from build123d import *

# Parameters (mm, degrees)
SKETCH025_W     = 41
SKETCH025_H     = 41
PAD017_DEPTH    = 22.6
SKETCH026_R     = 19.8
PAD018_DEPTH    = 12.6
SKETCH027_W     = 9
SKETCH027_H     = 4.7
POCKET007_DEPTH = 5


with BuildPart() as part:
    # Sketch025 → Pad017 (new body)
    with BuildSketch(Plane.XY):
        with Locations((3.199544, 3.041725)):
            Rectangle(SKETCH025_W, SKETCH025_H)
    extrude(amount=PAD017_DEPTH)

    # Sketch026 (on Face6 of Pad017) → Pad018 (join)
    with BuildSketch(Plane.XY.offset(22.6)):
        with Locations((3.297032, 2.892403)):
            Circle(SKETCH026_R)
    extrude(amount=PAD018_DEPTH)

    # Sketch027 (on Face3 of Pad018) → Pocket007 (cut)
    with BuildSketch(Plane.XZ.offset(17.458275)):
        with Locations((3.457133, 7.14271)):
            Rectangle(SKETCH027_W, SKETCH027_H)
    extrude(amount=-POCKET007_DEPTH, mode=Mode.SUBTRACT)


with BuildPart() as part_1:
    # Body006 placement: moved
    add(part.part.moved(Location((-5, 10, 65))))


solid = part_1.part
The model under review builds one solid part; all positions refer to its coordinate system, in mm. A direction names the side the tool comes from. Round coordinates to 2 decimals unless told otherwise and drop trailing zeros. Order: outer loops, then holes, each group sorted by start corner. A loop starts at its lowest first (then second) coordinate and runs counter-clockwise, first axis right, second up. Notation, with made-up numbers: (41, 76.25) -> (80, 76.25) arc R10 ccw to (80, 94.25) -> close; hole circle Ø1 at (4, 47.5). An arc over 180 degrees is marked (long way). Write item = value, one per line. Start each with the question number.
Item 1: Consider section C-C on x = 1.5. Write out the cut boundary in (y, z), plus the area to 3 significant figures.
Item 2: For line 1 along Z through (x, y) = (-4.5, -5); line 2 along Z through (x, y) = (17.5, 31); line 3 along Y through (x, z) = (-0.5, 73), list the stretches that pass through material, from the lowest coordinate up.
Item 3: Mouldability with a two-part tool opening along X and no side actions: class faces 4 (the face through (2.957, -5, 72)), 5 (the face through (-2, 13, 65)), 6 (the face through (18.7, 13, 76)) as released by +X, released by -X, zero draft, split by the parting line, or undercut.
Item 4: Clearance check with flat-ended pins moving along their axes: pin 1 Ø1.5 at (y, z) = (19, 88.5) entering from -X; pin 2 Ø1.5 at (x, z) = (-3.5, 93.5) entering from -Y; pin 3 Ø1 at (y, z) = (20, 88.5) entering from -X. State where each tip first meets the part, or that it passes through.
Item 5: Consider section A-A on z = 71. Write out the cut boundary in (x, y).
Item 6: Consider section B-B on y = 8.5. Write out the cut boundary in (x, z).
Item 7: Consider section D-D on z = 91. Write out the cut boundary in (x, y), plus the area to 3 significant figures.
Item 8: For faces 1 (the face through (-2, -5, 74.493)), 2 (the face through (-9.5, 31.4, 87.6)), 3 (the face through (-2, -7.458, 76)), list the 3-axis set-ups (+Z, -Z, +X, -X, +Y, -Y) from which the entire face can be reached by the end or side of a thin tool; tool diameter is ignored.
Conclusion:
q1.outline = (-7.46, 65) -> (33.54, 65) -> (33.54, 87.6) -> (32.43, 87.6) -> (32.43, 100.2) -> (-6.65, 100.2) -> (-6.65, 87.6) -> (-7.46, 87.6) -> (-7.46, 74.49) -> (-2.46, 74.49) -> (-2.46, 69.79) -> (-7.46, 69.79) -> close
q1.area = 1,400 mm2
q2.line_1 = 65 to 69.79, 74.49 to 100.2
q2.line_2 = 65 to 87.6
q2.line_3 = -2.46 to 33.54
q3.face_4 = undercut
q3.face_5 = zero draft
q3.face_6 = released by +X
q4.pin_1 = -20.76
q4.pin_2 = -6.88
q4.pin_3 = -20.37
q5.outline = (-22.3, -7.46) -> (-6.04, -7.46) -> (-6.04, -2.46) -> (2.96, -2.46) -> (2.96, -7.46) -> (18.7, -7.46) -> (18.7, 33.54) -> (-22.3, 33.54) -> close
q6.outline = (-22.3, 65) -> (18.7, 65) -> (18.7, 87.6) -> (17.6, 87.6) -> (17.6, 100.2) -> (-21.01, 100.2) -> (-21.01, 87.6) -> (-22.3, 87.6) -> close
q7.outline = circle Ø39.6 at (-1.7, 12.89)
q7.area = 1,230 mm2
q8.face_1 = -Y
q8.face_2 = +Z
q8.face_3 = +Z, -Z, +X, -X, -Y
